Here's the drawing with two shaded views (mm, measured from the low corner). I have some questions. Round coordinates to 2 decimals unless told otherwise and drop trailing zeros. Order: outer loops, then holes, each group sorted by start corner. A loop starts at its lowest first (then second) coordinate and runs counter-clockwise, first axis right, second up. Notation, with made-up numbers: (33.25, -17) -> (69.25, -17) arc R17 cw to (69.25, -1) -> close; hole circle Ø6 at (29, -15.5). An arc over 180 degrees is marked (long way). Answer in a Markdown table with one row per item.
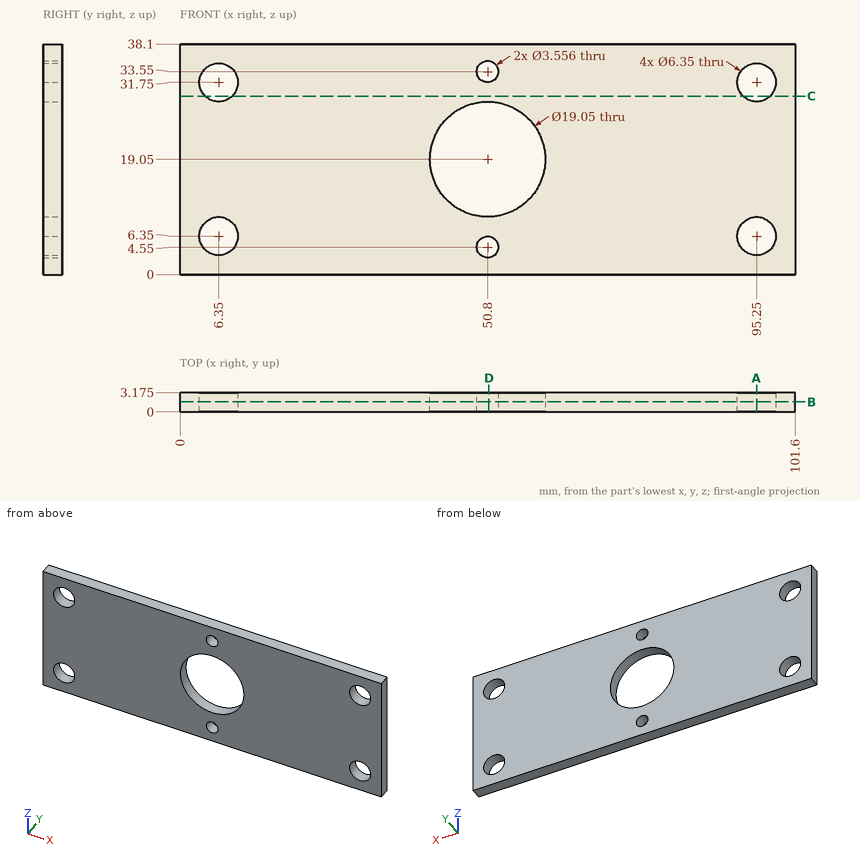
1. Please list where these lines run through material, in increasing order: line 1 along Z through (x, y) = (50.8, 1) (3 decimals); line 2 along Z through (x, y) = (95.25, 1.1) (3 decimals); line 3 along X through (y, z) = (3.05, 6.5).
Numbers:
| item | result |
|---|---|
| line 1 | z = 0 to 2.772, 6.328 to 9.525, 28.575 to 31.772, 35.328 to 38.1 |
| line 2 | z = 0 to 3.175, 9.525 to 28.575, 34.925 to 38.1 |
| line 3 | x = 0 to 3.18, 9.52 to 92.08, 98.42 to 101.6 |
2. Suppose I cut it at C-C on z = 29.5. Write out the boundary of the cut face in (x, y) (3 decimals), then the cut area to 3 significant figures.
Numbers:
| item | result |
|---|---|
| outline | (0, 0) -> (4.11, 0) -> (4.11, 3.175) -> (0, 3.175) -> close; (8.59, 0) -> (93.01, 0) -> (93.01, 3.175) -> (8.59, 3.175) -> close; (97.49, 0) -> (101.6, 0) -> (101.6, 3.175) -> (97.49, 3.175) -> close |
| area | 294 mm2 |
3. For pin 1 Ø3 at (x, z) = (72, 22) entering from -Y, with a flat end and sliding along its axis, tell me the tip position at first contact or that it passes through.
Numbers:
| item | result |
|---|---|
| pin 1 | stops at y = 0 |
4. Suppose I cut it at D-D on x = 51. Write out the boundary of the cut face in (y, z) (3 decimals).
Numbers:
| item | result |
|---|---|
| outline | (0, 0) -> (3.175, 0) -> (3.175, 2.783) -> (0, 2.783) -> close; (0, 6.317) -> (3.175, 6.317) -> (3.175, 9.527) -> (0, 9.527) -> close; (0, 28.573) -> (3.175, 28.573) -> (3.175, 31.783) -> (0, 31.783) -> close; (0, 35.317) -> (3.175, 35.317) -> (3.175, 38.1) -> (0, 38.1) -> close |
5. Suppose I cut it at B-B on y = 1.65. Write out the boundary of the cut face in (x, z) (3 decimals).
Numbers:
| item | result |
|---|---|
| outline | (0, 0) -> (101.6, 0) -> (101.6, 38.1) -> (0, 38.1) -> close; hole circle Ø6.35 at (6.35, 6.35); hole circle Ø6.35 at (6.35, 31.75); hole circle Ø19.05 at (50.8, 19.05); hole circle Ø3.556 at (50.8, 4.55); hole circle Ø3.556 at (50.8, 33.55); hole circle Ø6.35 at (95.25, 6.35); hole circle Ø6.35 at (95.25, 31.75) |
6. Suppose I cut it at A-A on x = 95.25. Write out the boundary of the cut face in (y, z) (3 decimals).
Numbers:
| item | result |
|---|---|
| outline | (0, 0) -> (3.175, 0) -> (3.175, 3.175) -> (0, 3.175) -> close; (0, 9.525) -> (3.175, 9.525) -> (3.175, 28.575) -> (0, 28.575) -> close; (0, 34.925) -> (3.175, 34.925) -> (3.175, 38.1) -> (0, 38.1) -> close |
